```python
from build123d import *

# Parameters (mm, degrees)
SKETCH1_W           = 7.937979337
SKETCH1_H           = 0.559115352
BOSS_EXTRUDE1_DEPTH = 11.5
SKETCH2_R           = 1.5
CUT_EXTRUDE1_DEPTH  = 8
CUT_EXTRUDE2_DEPTH  = 8
SKETCH4_R           = 2.5
CUT_EXTRUDE3_DEPTH  = 1.5


with BuildPart() as part:
    # Sketch1 → Boss-Extrude1 (new body)
    with BuildSketch(Plane(origin=(0, 0, 0), x_dir=(1, 0, 0), z_dir=(0, 1, 0))):
        with BuildLine():
            Line((-40.080884648, -36.23445276), (-40.080884648, 18.423402639))
            Line((-40.080884648, 18.423402639), (-40.64, 18.423402639))
            Line((-40.64, 18.423402639), (-40.64, -36.199115352))
            ThreePointArc((-40.64, -36.199115352), (-40.359884529, -36.207958509), (-40.080884648, -36.23445276))
        make_face()
        with BuildLine():
            Line((-40.080884648, 18.423402639), (-40.080884648, 36.23445276))
            ThreePointArc((-40.080884648, 36.23445276), (-40.359884529, 36.207958509), (-40.64, 36.199115352))
            Line((-40.64, 36.199115352), (-40.64, 18.423402639))
            Line((-40.64, 18.423402639), (-40.080884648, 18.423402639))
        make_face()
        with BuildLine():
            Line((-36.23445276, 40.080884648), (-7.937979337, 40.080884648))
            Line((-7.937979337, 40.080884648), (-7.937979337, 40.64))
            Line((-7.937979337, 40.64), (-36.199115352, 40.64))
            ThreePointArc((-36.199115352, 40.64), (-36.207958509, 40.359884529), (-36.23445276, 40.080884648))
        make_face()
        with BuildLine():
            Line((0, 40.64), (0, 40.080884648))
            Line((0, 40.080884648), (36.23445276, 40.080884648))
            ThreePointArc((36.23445276, 40.080884648), (36.207958509, 40.359884529), (36.199115352, 40.64))
            Line((36.199115352, 40.64), (0, 40.64))
        make_face()
        with Locations((-3.968989669, 40.360442324)):
            Rectangle(SKETCH1_W, SKETCH1_H)
        with BuildLine():
            ThreePointArc((40.64, 36.199115352), (40.359884529, 36.207958509), (40.080884648, 36.23445276))
            Line((40.080884648, 36.23445276), (40.080884648, 28.268480093))
            Line((40.080884648, 28.268480093), (40.64, 28.268480093))
            Line((40.64, 28.268480093), (40.64, 36.199115352))
        make_face()
        with BuildLine():
            Line((40.64, 28.268480093), (40.080884648, 28.268480093))
            Line((40.080884648, 28.268480093), (40.080884648, -36.23445276))
            ThreePointArc((40.080884648, -36.23445276), (40.359884529, -36.207958509), (40.64, -36.199115352))
            Line((40.64, -36.199115352), (40.64, 28.268480093))
        make_face()
        with BuildLine():
            ThreePointArc((40.64, -36.199115352), (40.359884529, -36.207958509), (40.080884648, -36.23445276))
            ThreePointArc((40.080884648, -36.23445276), (37.499820351, -37.499820351), (36.23445276, -40.080884648))
            ThreePointArc((36.23445276, -40.080884648), (36.207958509, -40.359884529), (36.199115352, -40.64))
            Line((36.199115352, -40.64), (40.64, -40.64))
            Line((40.64, -40.64), (40.64, -36.199115352))
        make_face()
        with BuildLine():
            ThreePointArc((45.080884648, -40.64), (43.780179649, -37.499820351), (40.64, -36.199115352))
            Line((40.64, -36.199115352), (40.64, -40.64))
            Line((40.64, -40.64), (36.199115352, -40.64))
            ThreePointArc((36.199115352, -40.64), (37.499820351, -43.780179649), (40.64, -45.080884648))
            ThreePointArc((40.64, -45.080884648), (43.780179649, -43.780179649), (45.080884648, -40.64))
        make_face()
        with BuildLine():
            ThreePointArc((36.199115352, -40.64), (36.207958509, -40.359884529), (36.23445276, -40.080884648))
            Line((36.23445276, -40.080884648), (27.085817246, -40.080884648))
            Line((27.085817246, -40.080884648), (27.085817246, -40.64))
            Line((27.085817246, -40.64), (36.199115352, -40.64))
        make_face()
        with BuildLine():
            Line((27.085817246, -40.080884648), (-36.23445276, -40.080884648))
            ThreePointArc((-36.23445276, -40.080884648), (-36.207958509, -40.359884529), (-36.199115352, -40.64))
            Line((-36.199115352, -40.64), (27.085817246, -40.64))
            Line((27.085817246, -40.64), (27.085817246, -40.080884648))
        make_face()
        with BuildLine():
            Line((-40.64, -40.64), (-40.64, -36.199115352))
            ThreePointArc((-40.64, -36.199115352), (-43.780179649, -37.499820351), (-45.080884648, -40.64))
            ThreePointArc((-45.080884648, -40.64), (-43.780179649, -43.780179649), (-40.64, -45.080884648))
            ThreePointArc((-40.64, -45.080884648), (-37.499820351, -43.780179649), (-36.199115352, -40.64))
            Line((-36.199115352, -40.64), (-40.64, -40.64))
        make_face()
        with BuildLine():
            ThreePointArc((-36.23445276, -40.080884648), (-37.499820351, -37.499820351), (-40.080884648, -36.23445276))
            ThreePointArc((-40.080884648, -36.23445276), (-40.359884529, -36.207958509), (-40.64, -36.199115352))
            Line((-40.64, -36.199115352), (-40.64, -40.64))
            Line((-40.64, -40.64), (-36.199115352, -40.64))
            ThreePointArc((-36.199115352, -40.64), (-36.207958509, -40.359884529), (-36.23445276, -40.080884648))
        make_face()
        with BuildLine():
            Line((27.085817246, -40.64), (-36.199115352, -40.64))
            ThreePointArc((-36.199115352, -40.64), (-37.499820351, -43.780179649), (-40.64, -45.080884648))
            Line((-40.64, -45.080884648), (27.085817246, -45.080884648))
            Line((27.085817246, -45.080884648), (27.085817246, -40.64))
        make_face()
        with BuildLine():
            Line((-40.64, -36.199115352), (-40.64, 18.423402639))
            Line((-40.64, 18.423402639), (-45.080884648, 18.423402639))
            Line((-45.080884648, 18.423402639), (-45.080884648, -40.64))
            ThreePointArc((-45.080884648, -40.64), (-43.780179649, -37.499820351), (-40.64, -36.199115352))
        make_face()
        with BuildLine():
            ThreePointArc((40.64, -45.080884648), (37.499820351, -43.780179649), (36.199115352, -40.64))
            Line((36.199115352, -40.64), (27.085817246, -40.64))
            Line((27.085817246, -40.64), (27.085817246, -45.080884648))
            Line((27.085817246, -45.080884648), (40.64, -45.080884648))
        make_face()
        with BuildLine():
            Line((45.080884648, 28.268480093), (40.64, 28.268480093))
            Line((40.64, 28.268480093), (40.64, -36.199115352))
            ThreePointArc((40.64, -36.199115352), (43.780179649, -37.499820351), (45.080884648, -40.64))
            Line((45.080884648, -40.64), (45.080884648, 28.268480093))
        make_face()
        with BuildLine():
            ThreePointArc((45.080884648, 40.64), (43.780179649, 37.499820351), (40.64, 36.199115352))
            Line((40.64, 36.199115352), (40.64, 28.268480093))
            Line((40.64, 28.268480093), (45.080884648, 28.268480093))
            Line((45.080884648, 28.268480093), (45.080884648, 40.64))
        make_face()
        with BuildLine():
            ThreePointArc((40.64, 45.080884648), (37.499820351, 43.780179649), (36.199115352, 40.64))
            Line((36.199115352, 40.64), (40.64, 40.64))
            Line((40.64, 40.64), (40.64, 36.199115352))
            ThreePointArc((40.64, 36.199115352), (43.780179649, 37.499820351), (45.080884648, 40.64))
            ThreePointArc((45.080884648, 40.64), (43.780179649, 43.780179649), (40.64, 45.080884648))
        make_face()
        with BuildLine():
            ThreePointArc((36.199115352, 40.64), (36.207958509, 40.359884529), (36.23445276, 40.080884648))
            ThreePointArc((36.23445276, 40.080884648), (37.499820351, 37.499820351), (40.080884648, 36.23445276))
            ThreePointArc((40.080884648, 36.23445276), (40.359884529, 36.207958509), (40.64, 36.199115352))
            Line((40.64, 36.199115352), (40.64, 40.64))
            Line((40.64, 40.64), (36.199115352, 40.64))
        make_face()
        with BuildLine():
            Line((-7.937979337, 40.64), (0, 40.64))
            Line((0, 40.64), (36.199115352, 40.64))
            ThreePointArc((36.199115352, 40.64), (37.499820351, 43.780179649), (40.64, 45.080884648))
            Line((40.64, 45.080884648), (-7.937979337, 45.080884648))
            Line((-7.937979337, 45.080884648), (-7.937979337, 40.64))
        make_face()
        with BuildLine():
            Line((-36.199115352, 40.64), (-7.937979337, 40.64))
            Line((-7.937979337, 40.64), (-7.937979337, 45.080884648))
            Line((-7.937979337, 45.080884648), (-40.64, 45.080884648))
            ThreePointArc((-40.64, 45.080884648), (-37.499820351, 43.780179649), (-36.199115352, 40.64))
        make_face()
        with BuildLine():
            Line((-40.64, 40.64), (-36.199115352, 40.64))
            ThreePointArc((-36.199115352, 40.64), (-37.499820351, 43.780179649), (-40.64, 45.080884648))
            ThreePointArc((-40.64, 45.080884648), (-43.780179649, 43.780179649), (-45.080884648, 40.64))
            ThreePointArc((-45.080884648, 40.64), (-43.780179649, 37.499820351), (-40.64, 36.199115352))
            Line((-40.64, 36.199115352), (-40.64, 40.64))
        make_face()
        with BuildLine():
            ThreePointArc((-40.080884648, 36.23445276), (-37.499820351, 37.499820351), (-36.23445276, 40.080884648))
            ThreePointArc((-36.23445276, 40.080884648), (-36.207958509, 40.359884529), (-36.199115352, 40.64))
            Line((-36.199115352, 40.64), (-40.64, 40.64))
            Line((-40.64, 40.64), (-40.64, 36.199115352))
            ThreePointArc((-40.64, 36.199115352), (-40.359884529, 36.207958509), (-40.080884648, 36.23445276))
        make_face()
        with BuildLine():
            Line((-40.64, 18.423402639), (-40.64, 36.199115352))
            ThreePointArc((-40.64, 36.199115352), (-43.780179649, 37.499820351), (-45.080884648, 40.64))
            Line((-45.080884648, 40.64), (-45.080884648, 18.423402639))
            Line((-45.080884648, 18.423402639), (-40.64, 18.423402639))
        make_face()
    extrude(amount=BOSS_EXTRUDE1_DEPTH)

    # Sketch2 → Cut-Extrude1 (cut)
    with BuildSketch(Plane(origin=(0, 11.5, 0), x_dir=(1, 0, 0), z_dir=(0, 1, 0))):
        with Locations((-40.64, 40.64)):
            Circle(SKETCH2_R)
        with Locations((40.64, 40.64)):
            Circle(SKETCH2_R)
        with Locations((40.64, -40.64)):
            Circle(SKETCH2_R)
        with Locations((-40.64, -40.64)):
            Circle(SKETCH2_R)
    extrude(amount=-CUT_EXTRUDE1_DEPTH, mode=Mode.SUBTRACT)

    # Sketch3 → Cut-Extrude2 (cut)
    with BuildSketch(Plane(origin=(45.080884648, 0, 0), x_dir=(0, 0, -1), z_dir=(1, 0, 0))):
        with BuildLine():
            Line((30.979, 9.5), (23.479, 9.5))
            ThreePointArc((23.479, 9.5), (22.064786438, 8.914213562), (21.479, 7.5))
            Line((21.479, 7.5), (21.479, 3))
            ThreePointArc((21.479, 3), (22.064786438, 1.585786438), (23.479, 1))
            Line((23.479, 1), (30.979, 1))
            ThreePointArc((30.979, 1), (32.393213562, 1.585786438), (32.979, 3))
            Line((32.979, 3), (32.979, 7.5))
            ThreePointArc((32.979, 7.5), (32.393213562, 8.914213562), (30.979, 9.5))
        make_face()
    extrude(amount=-CUT_EXTRUDE2_DEPTH, mode=Mode.SUBTRACT)

    # Sketch4 → Cut-Extrude3 (cut)
    with BuildSketch(Plane(origin=(0, 11.5, 0), x_dir=(1, 0, 0), z_dir=(0, 1, 0))):
        with Locations((-40.64, 40.64)):
            Circle(SKETCH4_R)
        with Locations((40.64, 40.64)):
            Circle(SKETCH4_R)
        with Locations((40.64, -40.64)):
            Circle(SKETCH4_R)
        with Locations((-40.64, -40.64)):
            Circle(SKETCH4_R)
    extrude(amount=-CUT_EXTRUDE3_DEPTH, mode=Mode.SUBTRACT)


solid = part.part
```
The listing builds one solid part. Answer for the finished solid, in the listing's coordinates (mm). A direction names the side the tool comes from. Round coordinates to 2 decimals unless told otherwise and drop trailing zeros. Write each loop counter-clockwise with the first axis right and the second up, starting at its lowest first coordinate (ties: lowest second). Pieces come first, ordered by that corner, then holes. Notation, with made-up numbers: (28, 8.25) -> (78, 8.25) arc R26 cw to (78, 27.25) -> close; hole circle Ø2 at (82, 37). An arc over 180 degrees is marked (long way). Write item = value, one per line.
1) Which of the six approach directions +Z, -Z, +X, -X, +Y, -Y give full straight-line access (tool end or side, diameter ignored) to faces 1 (the flat face through (43, 9.5, -27)), 2 (the cylindrical face through (39.45, 6.8, 41.55)), 3 (the cylindrical face through (37.5, 5.7, 37.5))?
Check values:
face_1 = +X
face_2 = +Y
face_3 = +Y, -Y
2) Straight lines are drawn through the part: line 1 along X through (y, z) = (10.4, -40.64); line 2 along Z through (x, y) = (40.64, 5.25). For each, find the intervals that lie inside material, in ascending order. Write a range as [from, to].
Check values:
line_1 = [-45.08, -43.14], [-38.14, 38.14], [43.14, 45.08]
line_2 = [-45.08, -42.14], [-39.14, -32.98], [-21.48, 39.14], [42.14, 45.08]
3) Section A-A on z = 22.5 is taken. Write down the section's boundary in (x, y), plus the area to 3 significant figures.
Check values:
outline = (-45.08, 0) -> (-40.08, 0) -> (-40.08, 11.5) -> (-45.08, 11.5) -> close; (40.08, 0) -> (45.08, 0) -> (45.08, 11.5) -> (40.08, 11.5) -> close
area = 115 mm²
4) Section C-C on y = 5 is taken. Write down the section's boundary in (x, z).
Check values:
outline = (-45.08, -40.64) arc R4.44 ccw to (-40.64, -45.08) -> (40.64, -45.08) arc R4.44 ccw to (45.08, -40.64) -> (45.08, -32.98) -> (40.08, -32.98) -> (40.08, -36.23) arc R4.44 ccw to (36.23, -40.08) -> (-36.23, -40.08) arc R4.44 ccw to (-40.08, -36.23) -> (-40.08, 36.23) arc R4.44 ccw to (-36.23, 40.08) -> (36.23, 40.08) arc R4.44 ccw to (40.08, 36.23) -> (40.08, -21.48) -> (45.08, -21.48) -> (45.08, 40.64) arc R4.44 ccw to (40.64, 45.08) -> (-40.64, 45.08) arc R4.44 ccw to (-45.08, 40.64) -> close; hole circle Ø3 at (-40.64, -40.64); hole circle Ø3 at (-40.64, 40.64); hole circle Ø3 at (40.64, -40.64); hole circle Ø3 at (40.64, 40.64)
5) Section B-B on x = -29.5 is taken. Write down the section's boundary in (y, z), plus the area to 3 significant figures.
Check values:
outline = (0, -45.08) -> (11.5, -45.08) -> (11.5, -40.08) -> (0, -40.08) -> close; (0, 40.08) -> (11.5, 40.08) -> (11.5, 45.08) -> (0, 45.08) -> close
area = 115 mm²
6) For a pull along Z with two mould halves and no side action, classify faces 4 (the cylindrical face through (38.8, 10.76, 38.95)), 5 (the cylindrical face through (43.75, 5.67, 43.81)), 6 (the cylindrical face through (43.81, 5.67, -43.75)) as released by +Z, released by -Z, zero draft, split by the parting line, or undercut.
Check values:
face_4 = undercut
face_5 = released by +Z
face_6 = released by -Z
7) Given pin 1 (1.5 mm diameter, centred on x = -41.5, z = -40.5, fed in from +Y); pin 2 (1.3 mm diameter, centred on x = 42.5, y = 5, fed in from -Z); pin 3 (2.5 mm diameter, centred on x = -40.64, z = 40.64, fed in from +Y); pin 4 (4 mm diameter, centred on x = -42, z = 40, fed in from +Y), each flat-ended and moving along its own axis, determine where each tip first touches the part or whether it passes through.
Check values:
pin_1 = 10
pin_2 = -44.91
pin_3 = 3.5
pin_4 = 11.5
